Autodesk Inventor part; units mm, degrees
ref_plane "YZ Plane" through (0, 0, 0) normal (1, 0, 0) x (0, 1, 0)
ref_plane "XZ Plane" through (0, 0, 0) normal (0, 1, 0) x (-1, 0, 0)
ref_plane "XY Plane" through (0, 0, 0) normal (0, 0, 1) x (1, 0, 0)
sketch "Sketch1" plane through (0, 0, 0) normal (0, 0, 1) x (1, 0, 0)
  circle A0 centre (0, 0) radius 4.699
  dimension "head_dia" = 9.398
extrude "Extrusion1" add sketch "Sketch1" along normal blind 2.286
sketch "Sketch2" plane through (0, 0, 2.286) normal (0, 0, 1) x (1, 0, 0)
  circle A0 centre (0, 0) radius 3.175
  dimension "d5" = 6.35
extrude "Extrusion2" add sketch "Sketch2" along normal blind 2.413
sketch "Sketch3" plane through (0, 0, 4.699) normal (0, 0, 1) x (1, 0, 0)
  circle A0 centre (0, 0) radius 1.4224
  dimension "d8" = 2.8448
extrude "Extrusion3" add sketch "Sketch3" along normal blind 7.112
thread "Thread1"
fillet "Fillet1" radius 0.127 1 edges at (-4.699, 0, 0)
fillet "Fillet2" radius 0.127 1 edges at (-4.699, 0, 2.286)
fillet "Fillet3" radius 0.127 1 edges at (-3.175, 0, 4.699)
properties part number "fastener_screw"
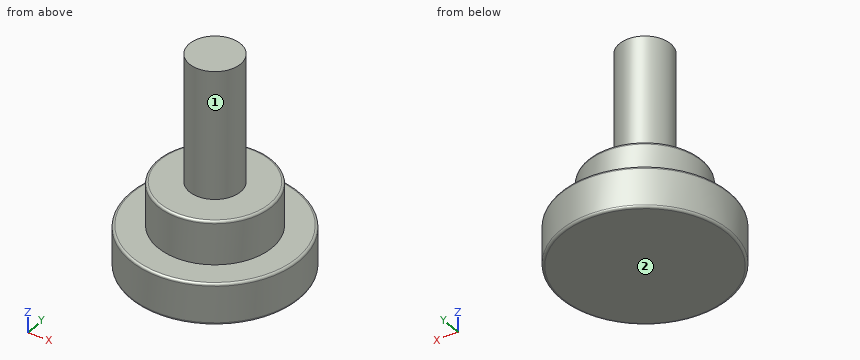
For this review, take the finished solid that the model builds, in its own axes (mm). Face numbers are marked on the shaded views. A direction names the side the tool comes from. Coordinates: 2 decimals unless noted, no trailing zeros. Write each loop counter-clockwise with the first axis right and the second up, starting at its lowest first coordinate (ties: lowest second). Pieces come first, ordered by that corner, then holes.
(1) Add section C-C on z = 1.25. Give the boundary of the cut face in (x, y), then the cut area to 3 significant figures.
(2) Add section D-D on z = 6. Give the boundary of the cut face in (x, y), then the cut area to 3 significant figures.
(3) Add section A-A on y = 0. Give the boundary of the cut face in (x, z) (3 decimals).
(4) Wall thickness on probe 1 along Z at (x, y) = (2.5, 1); probe 2 along Z at (x, y) = (-2, -2.75); probe 3 along Y at (x, z) = (-1.25, 9.5): over which ranges is each line inside the solid? List them lowest first.
(5) For pin 1 Ø2.5 at (x, y) = (-1, -2) entering from +Z; pin 2 Ø4 at (x, z) = (-1.5, 7) entering from -Y; pin 3 Ø1 at (y, z) = (1, 2) entering from -X; pin 4 Ø3 at (y, z) = (0, 5.5) entering from -X (3 decimals), all flat-tipped, find the tip position at first contact; note any pin that passes through.
(6) Tool access review of the marked faces 1 and 2: name each direction out of +Z, -Z, +X, -X, +Y, -Y from which nothing blocks a thin tool from reaching the whole face with its end or side.
Answer sheet:
1. outline: circle Ø9.4 at (0, 0)
1. area: 69.4 mm2
2. outline: circle Ø2.84 at (0, 0)
2. area: 6.36 mm2
3. outline: (-4.699, 0.127) arc R0.127 ccw to (-4.572, 0) - (4.572, 0) arc R0.127 ccw to (4.699, 0.127) - (4.699, 2.159) arc R0.127 ccw to (4.572, 2.286) - (3.175, 2.286) - (3.175, 4.572) arc R0.127 ccw to (3.048, 4.699) - (1.422, 4.699) - (1.422, 11.811) - (-1.422, 11.811) - (-1.422, 4.699) - (-3.048, 4.699) arc R0.127 ccw to (-3.175, 4.572) - (-3.175, 2.286) - (-4.572, 2.286) arc R0.127 ccw to (-4.699, 2.159) - close
4. probe 1: z = 0 to 4.7
4. probe 2: z = 0 to 2.29
4. probe 3: y = -0.68 to 0.68
5. pin 1: stops at z = 11.81
5. pin 2: stops at y = -1.42
5. pin 3: stops at x = -4.67
5. pin 4: stops at x = -3.175
6. face 1: +Z
6. face 2: -Z, +X, -X, +Y, -Y
